The drawing under review shows one solid part. Ordinate dimensions are in mm from its lowest x, y, z. Round coordinates to 2 decimals unless told otherwise and drop trailing zeros. Order: outer loops, then holes, each group sorted by start corner. A loop starts at its lowest first (then second) coordinate and runs counter-clockwise, first axis right, second up. Notation, with made-up numbers: M 56,-17 L 114,-17 A23 ccw 114,16 Z; hole C 29,58.5 d11. An arc over 180 degrees is marked long. Answer as a JSON object with one key per item and string values.
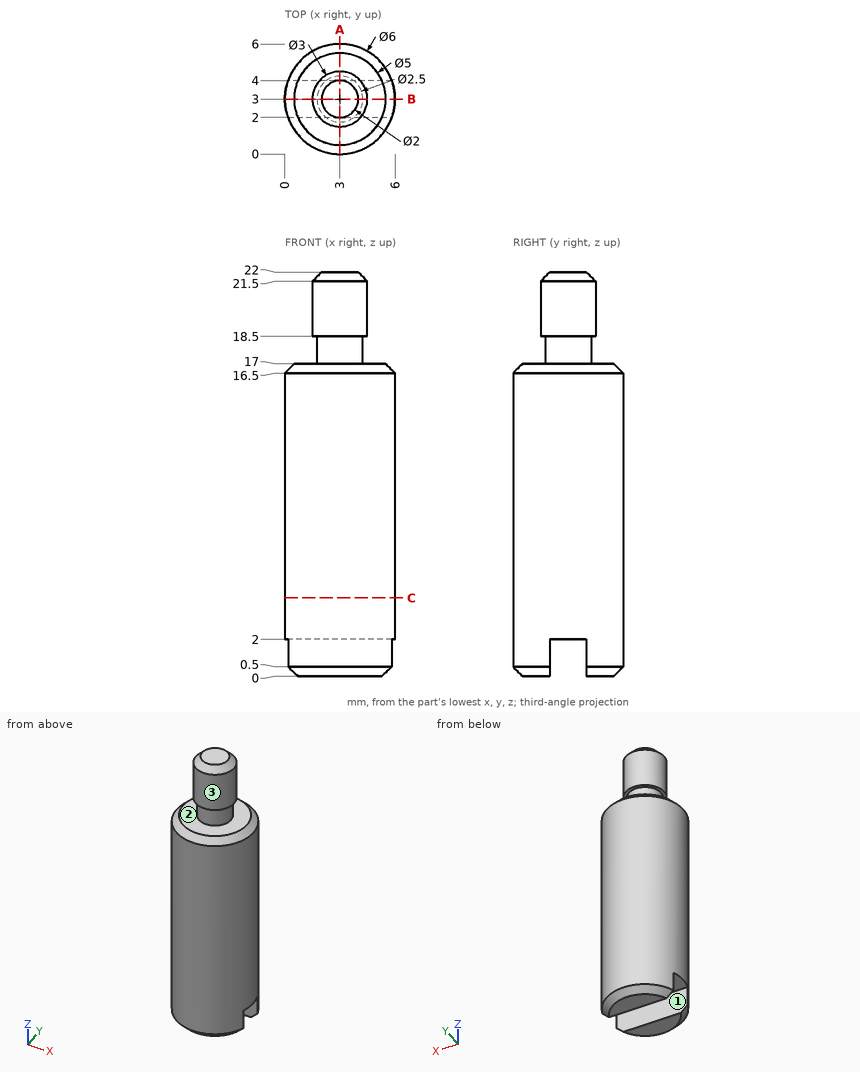
1) Add section C-C on z = 4.25. State the section outline as (x, y) points.
Geometry check:
{"outline": "C 3,3 d6"}
2) Insertion check: P1, Ø3, axis at x = 3, y = 1, coming from the +Z side; P2, Ø0.6, axis at x = 2.5, y = 3, coming from the -Z side; P3, Ø1.5, axis at x = 2, y = 4.5, coming from the +Z side; P4, Ø1, axis at x = 2, z = 1.5, coming from the +Y side. Each pin has a flat end and moves straight along its axis. Give the tip position at first contact, or say it passes through.
Geometry check:
{"P1": "stops at z = 22", "P2": "stops at z = 2", "P3": "stops at z = 21.95", "P4": "stops at y = 5.96"}
3) Add section B-B on y = 3. State the section outline as (x, z) points, and give its area (3 significant figures).
Geometry check:
{"outline": "M 0,2 L 6,2 L 6,16.5 L 5.5,17 L 4.25,17 L 4.25,18.5 L 4.5,18.5 L 4.5,21.5 L 4,22 L 2,22 L 1.5,21.5 L 1.5,18.5 L 1.75,18.5 L 1.75,17 L 0.5,17 L 0,16.5 Z", "area": "104 mm²"}
4) For L1, parallel to X at y = 0.4, z = 7.5; L2, parallel to X at y = 3.1, z = 11.5; L3, parallel to Z at x = 3.4, y = 1.35, list the stretches that pass through material, from the lowest coordinate up.
Geometry check:
{"L1": "x = 1.5 to 4.5", "L2": "x = 0 to 6", "L3": "z = 0 to 17"}
5) Mouldability with a two-part tool opening along Y and no side actions: class the marked faces 1, 2 and 3 as +Y half, -Y half, draft (parallel to the pull), parting line (faces both ways), or undercut.
Geometry check:
{"face 1": "undercut", "face 2": "draft", "face 3": "parting line"}
6) Add section A-A on x = 3. State the section outline as (y, z) points, and give its area (4 significant figures).
Geometry check:
{"outline": "M 0,0.5 L 0.5,0 L 2,0 L 2,2 L 4,2 L 4,0 L 5.5,0 L 6,0.5 L 6,16.5 L 5.5,17 L 4.25,17 L 4.25,18.5 L 4.5,18.5 L 4.5,21.5 L 4,22 L 2,22 L 1.5,21.5 L 1.5,18.5 L 1.75,18.5 L 1.75,17 L 0.5,17 L 0,16.5 Z", "area": "111.5 mm²"}
